from build123d import *

# Parameters (mm, degrees)
CUT_EXTRUDE1_REACH  = 3
BOSS_EXTRUDE1_DEPTH = 8


with BuildPart() as part:
    # Sketch1 → Revolve1 (revolve)
    with BuildSketch(Plane.XY):
        with BuildLine():
            Line((0, 0), (0, 8.5))
            ThreePointArc((0, 8.5), (1.767766953, 7.767766953), (2.5, 6))
            Line((2.5, 6), (2.5, 1))
            Line((2.5, 1), (3, 1))
            Line((3, 1), (3, 0))
            Line((3, 0), (0, 0))
        make_face()
    revolve(axis=Axis((0, 0, 0), (0, 1, 0)))

    # Sketch2 → Cut-Extrude1 (cut, up to next)
    with BuildSketch(Plane(origin=(0, 1, 0), x_dir=(1, 0, 0), z_dir=(0, 1, 0)), mode=Mode.PRIVATE) as cut_extrude1_sk1:
        with BuildLine():
            Line((2.5, 1.658312395), (2.5, -1.658312395))
            ThreePointArc((2.5, -1.658312395), (3, 0), (2.5, 1.658312395))
        make_face()
    cut_extrude1_tool1 = extrude(cut_extrude1_sk1.sketch, amount=-CUT_EXTRUDE1_REACH, mode=Mode.PRIVATE) & part.part
    add(cut_extrude1_tool1.solids().sort_by_distance((2.701501, 1, 0))[0], mode=Mode.SUBTRACT)

    # Sketch3 → Boss-Extrude1 (add)
    with BuildSketch(Plane.XZ):
        with BuildLine():
            Line((1.1, 1.4), (1.1, -1.4))
            ThreePointArc((1.1, -1.4), (0, -2.5), (-1.1, -1.4))
            Line((-1.1, -1.4), (-1.1, 1.4))
            ThreePointArc((-1.1, 1.4), (0, 2.5), (1.1, 1.4))
        make_face()
    extrude(amount=BOSS_EXTRUDE1_DEPTH)


solid = part.part
Can you work these out from the model? Positions are in its coordinate system, mm. A direction names the side the tool comes from. Give positions to 0.01 mm unless a question says otherwise; leave off trailing zeros. Loops run counter-clockwise (first coordinate to the right, second up) from the corner with the lowest first, then second, coordinate; pieces in that order, holes last. Notation, with made-up numbers: M 78.25,-22.5 L 136.25,-22.5 A30 cw 136.25,15.5 Z; hole C -28.5,15.25 d6. An arc over 180 degrees is marked long. One line per item, written item: value.
1) Imagine slicing it at A-A on x = 0. Write out the boundary of the cut face in (y, z), and give its area (3 significant figures).
Geometry check:
outline: M -8,-2.5 L 0,-2.5 L 0,-3 L 1,-3 L 1,-2.5 L 6,-2.5 A2.5 ccw 6,2.5 L 1,2.5 L 1,3 L 0,3 L 0,2.5 L -8,2.5 Z
area: 80.8 mm²
2) I'm going to push flat-ended pins straight in: pin 1 (1.4 mm diameter, centred on y = -5.5, z = 0, fed in from -X); pin 2 (1 mm diameter, centred on x = -2, y = 3.5, fed in from +Z); pin 3 (1.4 mm diameter, centred on y = -2, z = -0.5, fed in from +X). Where does each tip first touch, or does it pass through?
Geometry check:
pin 1: stops at x = -1.1
pin 2: stops at z = 2
pin 3: stops at x = 1.1
3) Imagine slicing it at D-D on x = -2.2. Write out the boundary of the cut face in (y, z).
Geometry check:
outline: M 0,-2.04 L 1,-2.04 L 1,-1.19 L 6,-1.19 A1.19 ccw 6,1.19 L 1,1.19 L 1,2.04 L 0,2.04 Z
4) Please list where these lines run through material, in increasing order: line 1 (Y direction, x = 2, z = -1.8); line 2 (X direction, y = -3, z = 1); line 3 (Z direction, x = 0.85, y = -1.25).
Geometry check:
line 1: y = 0 to 1
line 2: x = -1.1 to 1.1
line 3: z = -2.1 to 2.1
5) On a 3-axis mill with a long thin cutter (end or side, diameter ignored), from which of +Z, -Z, +X, -X, +Y, -Y can I reach the whole of each face in a straight line? I mean faces 1 (the face through (-0.54, 3.46, 2.44)), 2 (the face through (-1.1, -4, 0)), 3 (the face through (0, -3.9, -2.5)), 4 (the face through (1.1, -4, 0)). Say none if no direction works.
Geometry check:
face 1: +Y
face 2: +Z, -Z, -X, -Y
face 3: -Z, -Y
face 4: +Z, -Z, +X, -Y
6) Imagine slicing it at C-C on y = -1.5. Write out the boundary of the cut face in (x, z), and give its area (3 significant figures).
Geometry check:
outline: M -1.1,-1.4 A1.1 ccw 1.1,-1.4 L 1.1,1.4 A1.1 ccw -1.1,1.4 Z
area: 9.96 mm²
7) Imagine slicing it at B-B on z = -0.45. Write out the boundary of the cut face in (x, y), and give its area (3 significant figures).
Geometry check:
outline: M -2.97,0 L -1.1,0 L -1.1,-8 L 1.1,-8 L 1.1,0 L 2.5,0 L 2.5,1 L 2.46,1 L 2.46,6 A2.46 ccw -2.46,6 L -2.46,1 L -2.97,1 Z
area: 57.2 mm²
